Read the model definition and answer for the solid it produces. Units are mm, in the model's axes. A direction names the side the tool comes from. Coordinates: 2 decimals unless noted, no trailing zeros. Order: outer loops, then holes, each group sorted by start corner. A loop starts at its lowest first (then second) coordinate and runs counter-clockwise, first axis right, second up.
```python
from build123d import *

# Parameters (mm, degrees)
BOSS_EXTRUDE1_DEPTH = 2
SKETCH2_R           = 0.15
CUT_EXTRUDE1_DEPTH  = 3
SKETCH3_R           = 0.15
CUT_EXTRUDE4_DEPTH  = 3
FILLET2_R           = 1
FILLET3_R           = 1
SCALE2_SCALE        = 10


with BuildPart() as part:
    # Sketch1 → Boss-Extrude1 (new body)
    with BuildSketch(Plane.XY):
        with BuildLine():
            Line((-1.517184845, 0.342990579), (2.482815155, 0.342990579))
            ThreePointArc((2.482815155, 0.342990579), (6.442613129, -1.297211446), (8.082815155, -5.257009421))
            ThreePointArc((8.082815155, -5.257009421), (7.70871156, -7.378656338), (6.631523189, -9.244401325))
            Line((6.631523189, -9.244401325), (2.315107728, -5.50575471))
            ThreePointArc((2.315107728, -5.50575471), (2.262391387, -5.108396746), (2.650522581, -5.008264131))
            Line((2.650522581, -5.008264131), (6.955903492, -7.209487065))
            ThreePointArc((6.955903492, -7.209487065), (6.513613709, -2.574091852), (2.482815155, -0.242746306))
            Line((2.482815155, -0.242746306), (-1.517184845, -0.242746306))
            ThreePointArc((-1.517184845, -0.242746306), (-1.810053288, 0.050122136), (-1.517184845, 0.342990579))
        make_face()
    extrude(amount=BOSS_EXTRUDE1_DEPTH)

    # Sketch2 → Cut-Extrude1 (cut, through all)
    with BuildSketch(Plane(origin=(0, 0, 0), x_dir=(-1, 0, 0), z_dir=(0, 0, -1))):
        with Locations((-2.512956146, -5.277330883)):
            Circle(SKETCH2_R)
    extrude(amount=-CUT_EXTRUDE1_DEPTH, mode=Mode.SUBTRACT)

    # Sketch3 → Cut-Extrude4 (cut, through all)
    with BuildSketch(Plane(origin=(0, 0, 0), x_dir=(-1, 0, 0), z_dir=(0, 0, -1))):
        with Locations((1.517184845, 0.050122136)):
            Circle(SKETCH3_R)
    extrude(amount=-CUT_EXTRUDE4_DEPTH, mode=Mode.SUBTRACT)

    # Fillet2
    fillet2_edges = [part.edges().sort_by_distance(p)[0] for p in [
        (6.631523189, -9.244401325, 1),
    ]]
    fillet(fillet2_edges, radius=FILLET2_R)

    # Fillet3
    fillet3_edges = [part.edges().sort_by_distance(p)[0] for p in [
        (6.955903492, -7.209487065, 1),
    ]]
    fillet(fillet3_edges, radius=FILLET3_R)


with BuildPart() as part_1:
    # Scale2: scaled about (5.037716687, -4.281654958, 1)
    add(part.part.scale(SCALE2_SCALE).moved(Location((-45.339450183, 38.534894622, -9))))


solid = part_1.part
```
1) Determine the mould class of faces 1 (the flat face through (-10, -17, -9)), 2 (the cylindrical face through (22.275, -27.816, 1.14)), 3 (the cylindrical face through (33.604, -29.212, 0.86)), 4 (the cylindrical face through (-20.01, -12.75, 0.86)) for opening direction X: pulls with the +X half, pulls with the -X half, needs draft (parallel to the pull), parting line crosses it, or undercut.
A:
face 1: needs draft
face 2: undercut
face 3: pulls with the +X half
face 4: undercut
2) A cutting plane is placed at B-B, the plane x = -16.5. Determine the outline of the cut face in (y, z), and give its area (3 significant figures).
A:
outline: (-21.45, -9) - (-12.74, -9) - (-12.74, 11) - (-21.45, 11) - close; (35.75, -9) - (41.82, -9) - (41.82, 11) - (35.75, 11) - close
area: 296 mm2
3) Which of the six approach directions +Z, -Z, +X, -X, +Y, -Y give full straight-line access (tool end or side, diameter ignored) to faces 5 (the flat face through (-10, -17, 11)), 6 (the flat face through (-3.1, -19.59, 0.86))?
A:
face 5: +Z, +X, -X, +Y, -Y
face 6: +Z, -Z
4) Straight lines are drawn through the part: line 1 (Y direction, x = -19, z = -7.5); line 2 (Y direction, x = -26, z = -1.75); line 3 (Y direction, x = 18.5, z = -8). For each, find the intervals that lie inside material, in ascending order.
A:
line 1: y = -19.28 to -15.13, -13.35 to -11.47, 36.01 to 41.94
line 2: y = 36.11 to 41.96
line 3: y = -49.03 to -28.92, 14.72 to 26.14
5) A cutting plane is placed at D-D, the plane x = -32. Determine the outline of the cut face in (y, z), and give its area (3 significant figures).
A:
outline: (36.11, -9) - (41.96, -9) - (41.96, 11) - (36.11, 11) - close
area: 117 mm2
6) A cutting plane is placed at A-A, the plane y = -24. Determine the outline of the cut face in (x, z).
A:
outline: (-13.56, -9) - (5.52, -9) - (5.52, 11) - (-13.56, 11) - close; (26.27, -9) - (34.68, -9) - (34.68, 11) - (26.27, 11) - close
7) A cutting plane is placed at C-C, the plane z = 7.5. Determine the outline of the cut face in (x, y).
A:
outline: (-60.51, 36.11) - (-20.51, 36.11) arc R50.84 cw to (27.58, -20.01) arc R10 cw to (13.08, -27.86) - (-18.83, -11.55) arc R3.02 ccw to (-22.19, -16.52) - (12.54, -46.6) arc R10 ccw to (27.85, -43.85) arc R62.03 ccw to (35.49, -14.04) arc R56 ccw to (-20.51, 41.96) - (-60.51, 41.96) arc R2.93 ccw to start; hole circle Ø3 at (-60.51, 39.04); hole circle Ø3 at (-20.21, -14.24)
8) Flat-ended cylindrical pins translate along their axes: pin 1 Ø10 at (x, z) = (1.5, 0) entering from +Y; pin 2 Ø6 at (y, z) = (-39.5, 7) entering from +X; pin 3 Ø1.8 at (x, y) = (-20.21, -14.24) entering from -Z; pin 4 Ø5 at (y, z) = (-1, -3) entering from +X. Find the tip coordinate at first contact, or state that the pin passes through.
A:
pin 1: stops at y = 39.32
pin 2: stops at x = 31.28
pin 3: passes through
pin 4: stops at x = 34.49
